from build123d import *

# Parameters (mm, degrees)
SKETCH1_W               = 70
SKETCH1_H               = 45
BOSS_EXTRUDE1_DEPTH     = 1.6
SKETCH2_R               = 1.75
CUT_EXTRUDE1_DEPTH      = 42.639044177
MIRROR2_COPY_1_SKETCH_R = 1.75
MIRROR2_COPY_1_DEPTH    = 42.639044177


with BuildPart() as part:
    # Sketch1 → Boss-Extrude1 (new body)
    with BuildSketch(Plane.XY):
        Rectangle(SKETCH1_W, SKETCH1_H)
    extrude(amount=BOSS_EXTRUDE1_DEPTH)

    # Sketch2 → Cut-Extrude1 (cut, through all)
    with BuildSketch(Plane.XY.offset(1.6)):
        with Locations((-32, 19.5)):
            Circle(SKETCH2_R)
    cut_extrude1 = extrude(amount=-CUT_EXTRUDE1_DEPTH, mode=Mode.SUBTRACT)

    # Mirror1: Cut-Extrude1 across plane
    add(cut_extrude1.mirror(Plane.ZX), mode=Mode.SUBTRACT)

    # Mirror2: Cut-Extrude1 across plane
    add(cut_extrude1.mirror(Plane(origin=(0, 0, 0), x_dir=(0, 0, 1), z_dir=(1, 0, 0))), mode=Mode.SUBTRACT)

    # Mirror2 copy 1 sketch → Mirror2 copy 1 (cut, through all)
    with BuildSketch(Plane(origin=(0, 0, 1.6), x_dir=(-1, 0, 0), z_dir=(0, 0, 1))):
        with Locations((-32, 19.5)):
            Circle(MIRROR2_COPY_1_SKETCH_R)
    extrude(amount=-MIRROR2_COPY_1_DEPTH, mode=Mode.SUBTRACT)


solid = part.part
The listing builds one solid part. Answer for the finished solid, in the listing's coordinates (mm). Coordinates: 2 decimals unless noted, no trailing zeros. Write each loop counter-clockwise with the first axis right and the second up, starting at its lowest first coordinate (ties: lowest second). Pieces come first, ordered by that corner, then holes. Notation, with made-up numbers: (-18.5, 15.5) -> (17.5, 15.5) arc R21 ccw to (17.5, 51.5) -> close; hole circle Ø5 at (-4, 10). An arc over 180 degrees is marked (long way). One line per question, with ' | ' between items.
1. Straight lines are drawn through the part: line 1 (Y direction, x = -32, z = 1.2); line 2 (X direction, y = -19.5, z = 0.75); line 3 (X direction, y = -18, z = 1.45). For each, find the intervals that lie inside material, in ascending order.
Verdict:
line 1: y = -22.5 to -21.25, -17.75 to 17.75, 21.25 to 22.5 | line 2: x = -35 to -33.75, -30.25 to 30.25, 33.75 to 35 | line 3: x = -35 to -32.9, -31.1 to 31.1, 32.9 to 35
2. For a pull along Y with two mould halves and no side action, classify faces 1 (the flat face through (0, -22.5, 1)), 2 (the flat face through (-35, 0, 1)), 3 (the cylindrical face through (-33.29, 20.68, 0.81)), 4 (the flat face through (0, 22.5, 1)) as released by +Y, released by -Y, zero draft, split by the parting line, or undercut.
Verdict:
face 1: released by -Y | face 2: zero draft | face 3: undercut | face 4: released by +Y
3. Section A-A (y = 19.5) is taken. Determine the outline of the cut face in (x, z), and give its area (3 significant figures).
Verdict:
outline: (-35, 0) -> (-33.75, 0) -> (-33.75, 1.6) -> (-35, 1.6) -> close; (-30.25, 0) -> (30.25, 0) -> (30.25, 1.6) -> (-30.25, 1.6) -> close; (33.75, 0) -> (35, 0) -> (35, 1.6) -> (33.75, 1.6) -> close | area: 101 mm^2
4. Section B-B (x = -32) is taken. Determine the outline of the cut face in (y, z), and give its area (3 significant figures).
Verdict:
outline: (-22.5, 0) -> (-21.25, 0) -> (-21.25, 1.6) -> (-22.5, 1.6) -> close; (-17.75, 0) -> (17.75, 0) -> (17.75, 1.6) -> (-17.75, 1.6) -> close; (21.25, 0) -> (22.5, 0) -> (22.5, 1.6) -> (21.25, 1.6) -> close | area: 60.8 mm^2
